Autodesk Inventor part; units mm, degrees
ref_plane "YZ Plane" through (0, 0, 0) normal (1, 0, 0) x (0, 1, 0)
ref_plane "XZ Plane" through (0, 0, 0) normal (0, 1, 0) x (-1, 0, 0)
ref_plane "XY Plane" through (0, 0, 0) normal (0, 0, 1) x (1, 0, 0)
sketch "Esquisse1" plane through (0, 0, 0) normal (0, 0, 1) x (1, 0, 0)
  line L0 (-141.642, 40.418) -> (158.358, 40.418)
  line L1 (158.358, 40.418) -> (158.358, -24.582)
  line L2 (158.358, -24.582) -> (-141.642, -24.582)
  line L3 (-141.642, -24.582) -> (-141.642, 40.418)
  point P0 (0, 0)
  dimension "d0" = 300
  dimension "d1" = 65
extrude "Extrusion1" add sketch "Esquisse1" along normal blind 4
sketch "Esquisse2" plane through (0, 0, 4) normal (0, 0, 1) x (1, 0, 0)
  line L0 (-141.642, -24.582) -> (158.358, -24.582)
  line L1 (-138.642, 12.418) -> (-111.642, 12.418)
  line L2 (-111.642, 12.418) -> (-111.642, -24.582)
  line L3 (-111.642, -24.582) -> (-138.642, -24.582)
  line L4 (-138.642, -24.582) -> (-138.642, 12.418)
  line L5 (128.358, 12.418) -> (155.358, 12.418)
  line L6 (155.358, 12.418) -> (155.358, -24.582)
  line L7 (155.358, -24.582) -> (128.358, -24.582)
  line L8 (128.358, -24.582) -> (128.358, 12.418)
  line L9 (158.358, -24.582) -> (158.358, 40.418)
  line L10 (-141.642, 40.418) -> (-141.642, -24.582)
  point P0 (0, 0)
  dimension "d34" = 270
  dimension "d36" = 270
  dimension "d37" = 27
  dimension "d38" = 27
  dimension "d39" = 0
  dimension "d40" = 0
  dimension "d41" = 37
extrude "Extrusion2" add sketch "Esquisse2" along normal blind 30
sketch "Esquisse3" plane through (0, 0, 0) normal (0, 0, -1) x (-1, 0, 0)
  line L0 (-148.358, 35.418) -> (131.642, 35.418)
  line L1 (131.642, 35.418) -> (131.642, 25.418)
  line L2 (131.642, 25.418) -> (-148.358, 25.418)
  line L3 (-148.358, 25.418) -> (-148.358, 35.418)
  line L4 (-148.358, 20.418) -> (131.642, 20.418)
  line L5 (131.642, 20.418) -> (131.642, 10.418)
  line L6 (131.642, 10.418) -> (-148.358, 10.418)
  line L7 (-148.358, 10.418) -> (-148.358, 20.418)
  line L8 (-158.358, 40.418) -> (141.642, 40.418)
  line L9 (-148.358, 5.418) -> (131.642, 5.418)
  line L10 (131.642, 5.418) -> (131.642, -4.582)
  line L11 (131.642, -4.582) -> (-148.358, -4.582)
  line L12 (-148.358, -4.582) -> (-148.358, 5.418)
  line L13 (-148.358, -9.582) -> (131.642, -9.582)
  line L14 (131.642, -9.582) -> (131.642, -19.582)
  line L15 (131.642, -19.582) -> (-148.358, -19.582)
  line L16 (-148.358, -19.582) -> (-148.358, -9.582)
  line L17 (141.642, -24.582) -> (-158.358, -24.582)
  line L18 (-158.358, -24.582) -> (-158.358, 40.418)
  dimension "d14" = 5
  dimension "d15" = 10
  dimension "d16" = 5
  dimension "d17" = 10
  dimension "d20" = 5
  dimension "d21" = 10
  dimension "d22" = 5
  dimension "d23" = 10
  dimension "d24" = 280
  dimension "d25" = 280
  dimension "d26" = 280
  dimension "d27" = 280
  dimension "d28" = 10
  dimension "d29" = 10
  dimension "d30" = 10
  dimension "d31" = 10
extrude "Extrusion3" cut sketch "Esquisse3" against normal blind 1
sketch "Esquisse4" plane through (0, 0, 4) normal (0, 0, 1) x (1, 0, 0)
  line L0 (-16.642, 20.418) -> (33.358, 20.418)
  line L1 (33.358, 20.418) -> (33.358, 17.418)
  line L2 (33.358, 17.418) -> (-16.642, 17.418)
  line L3 (-16.642, 17.418) -> (-16.642, 20.418)
  line L4 (-111.642, -24.582) -> (128.358, -24.582)
  line L5 (158.358, -24.582) -> (158.358, 40.418)
  point P0 (0, 0)
  dimension "d42" = 42
  dimension "d43" = 3
  dimension "d44" = 50
  dimension "d45" = 125
extrude "Extrusion4" add sketch "Esquisse4" along normal blind 30
properties part number "pièce_chassis"
Can you work these out from the model? Positions are in its coordinate system, mm. A direction names the side the tool comes from. Round coordinates to 2 decimals unless told otherwise and drop trailing zeros. Order: outer loops, then holes, each group sorted by start corner. A loop starts at its lowest first (then second) coordinate and runs counter-clockwise, first axis right, second up.
(1) I'm going to push flat-ended pins straight in: pin 1 (3 mm diameter, centred on x = 111, y = -12.5, fed in from +Z); pin 2 (1 mm diameter, centred on x = 57, y = 13.5, fed in from -Z); pin 3 (8 mm diameter, centred on x = 6, z = 17, fed in from -Y). Where does each tip first touch, or does it pass through?
Results are:
pin 1: stops at z = 4
pin 2: stops at z = 1
pin 3: stops at y = 17.42
(2) If we section it at C-C (x = -42): Please give me the cut outline in (y, z), plus the area to 3 significant figures.
Results are:
outline: (-24.58, 0) - (-19.58, 0) - (-19.58, 1) - (-9.58, 1) - (-9.58, 0) - (-4.58, 0) - (-4.58, 1) - (5.42, 1) - (5.42, 0) - (10.42, 0) - (10.42, 1) - (20.42, 1) - (20.42, 0) - (25.42, 0) - (25.42, 1) - (35.42, 1) - (35.42, 0) - (40.42, 0) - (40.42, 4) - (-24.58, 4) - close
area: 220 mm2
(3) We'd pull the mould along X, two halves only. Please class faces 1 (the face through (6, 8, 0)), 2 (the face through (155.358, -6, 19)), 3 (the face through (128.358, -6, 19)): +X half, -X half, draft (parallel to the pull), parting line (faces both ways), or undercut.
Results are:
face 1: draft
face 2: +X half
face 3: undercut
(4) If we section it at A-A (z = 10): Please give me the cut outline in (x, y), plus the area to 3 significant figures.
Results are:
outline: (-138.64, -24.58) - (-111.64, -24.58) - (-111.64, 12.42) - (-138.64, 12.42) - close; (-16.64, 17.42) - (33.36, 17.42) - (33.36, 20.42) - (-16.64, 20.42) - close; (128.36, -24.58) - (155.36, -24.58) - (155.36, 12.42) - (128.36, 12.42) - close
area: 2,150 mm2
(5) If I drill on L1, parallel to X at y = 10, z = 5.5; L2, parallel to Z at x = 87, y = 2; L3, parallel to Z at x = 100, y = 23, over which ranges is the centre line in solid material (lowest first)?
Results are:
L1: x = -138.64 to -111.64, 128.36 to 155.36
L2: z = 1 to 4
L3: z = 0 to 4
(6) If we section it at D-D (y = -14): Please give me the cut outline in (x, z), plus the area to 3 significant figures.
Results are:
outline: (-141.64, 0) - (-131.64, 0) - (-131.64, 1) - (148.36, 1) - (148.36, 0) - (158.36, 0) - (158.36, 4) - (155.36, 4) - (155.36, 34) - (128.36, 34) - (128.36, 4) - (-111.64, 4) - (-111.64, 34) - (-138.64, 34) - (-138.64, 4) - (-141.64, 4) - close
area: 2,540 mm2
(7) On a 3-axis mill with a long thin cutter (end or side, diameter ignored), from which of +Z, -Z, +X, -X, +Y, -Y can I reach the whole of each face in a straight line? I mean faces 4 (the face through (-111.642, -6, 19)), 5 (the face through (-138.642, -6, 19)), 6 (the face through (10, 15, 1)). Say none if no direction works.
Results are:
face 4: +Z, +Y, -Y
face 5: +Z, -X, +Y, -Y
face 6: -Z
(8) If we section it at B-B (y = 28.5): Please give me the cut outline in (x, z), plus the area to 3 significant figures.
Results are:
outline: (-141.64, 0) - (-131.64, 0) - (-131.64, 1) - (148.36, 1) - (148.36, 0) - (158.36, 0) - (158.36, 4) - (-141.64, 4) - close
area: 920 mm2
